```python
from build123d import *

# Parameters (mm, degrees)
F0_R     = 1.294923
F1_DEPTH = 2
F2_W     = 10
F2_H     = 37.403586
F3_DEPTH = 25
F4_W     = 2.4
F4_H     = 37.403586
F5_DEPTH = 20
F6_R     = 1
F7_DEPTH = 25


with BuildPart() as f1:
    # F0 (on Front) → F1 (new body)
    with BuildSketch(Plane.XZ):
        Polygon((23.701793, 0), (0, 23.701793), (-23.701793, 0), (0, -23.701793), align=None)
        with Locations((0, -8)):
            Circle(F0_R, mode=Mode.SUBTRACT)
        with Locations((-8, 0)):
            Circle(F0_R, mode=Mode.SUBTRACT)
        with Locations((8, 0)):
            Circle(F0_R, mode=Mode.SUBTRACT)
        with Locations((0, 8)):
            Circle(F0_R, mode=Mode.SUBTRACT)
    extrude(amount=F1_DEPTH)

    # F2 (on face) → F3 (join)
    with BuildSketch(Plane(origin=(0, 0, 0), x_dir=(-1, 0, 0), z_dir=(0, 1, 0))):
        Rectangle(F2_W, F2_H)
    extrude(amount=F3_DEPTH)

    # F4 (on face) → F5 (cut)
    with BuildSketch(Plane(origin=(0, 25, 0), x_dir=(-1, 0, 0), z_dir=(0, 1, 0))):
        Rectangle(F4_W, F4_H)
    extrude(amount=-F5_DEPTH, mode=Mode.SUBTRACT)

    # F6 (on face) → F7 (cut)
    with BuildSketch(Plane(origin=(-5, 0, 0), x_dir=(0, -1, 0), z_dir=(-1, 0, 0))):
        with Locations((-20, 10)):
            Circle(F6_R)
        with Locations((-10, 10)):
            Circle(F6_R)
        with Locations((-10, 0)):
            Circle(F6_R)
        with Locations((-20, 0)):
            Circle(F6_R)
        with Locations((-20, -10)):
            Circle(F6_R)
        with Locations((-10, -10)):
            Circle(F6_R)
    extrude(amount=-F7_DEPTH, mode=Mode.SUBTRACT)


solid = f1.part
```
The listing builds one solid part. Answer for the finished solid, in the listing's coordinates (mm). A direction names the side the tool comes from. Give positions to 0.01 mm unless a question says otherwise; leave off trailing zeros. Order: outer loops, then holes, each group sorted by start corner. A loop starts at its lowest first (then second) coordinate and runs counter-clockwise, first axis right, second up. Notation, with made-up numbers: M 57,35 L 98,35 A18 ccw 98,42 Z; hole C 15,-19 d9. An arc over 180 degrees is marked long. Put each result on its own line as item: value. Start each with the question number.
Item 1: Which of the six approach directions +Z, -Z, +X, -X, +Y, -Y give full straight-line access (tool end or side, diameter ignored) to faces 4 (the face through (2, 12, -18.702)), 5 (the face through (-0.169, -0.986, 9.284)), 6 (the face through (-3.127, 20.737, -9.324)), 7 (the face through (5, 12, 0)), 8 (the face through (2, 12, 18.702))?
Item 2: The part is cut by section C-C, the plane z = 10. Determine the outline of the cut face in (x, y).
Item 3: For a pull along X with two mould halves and no side action, classify faces 1 (the face through (0, -2, 0)), 2 (the face through (-1.2, 15, 0)), 3 (the face through (-12, -1, -11.7)) as +X half, -X half, draft (parallel to the pull), parting line (faces both ways), or undercut.
Item 4: The part is cut by section A-A, the plane y = 20. State how many separate pieces and enclosed holes the cut face has, and give its area (3 significant figures).
Item 5: The part is cut by section B-B, the plane y = 7. Determine the outline of the cut face in (x, z).
Item 6: The part is cut by section D-D, the plane x = 4. Determine the outline of the cut face in (y, z), and give its area (3 significant figures).
Item 7: Find the intervals of material crossed by line 1 along Z through (x, y) = (3.6, 10); line 2 along X through (y, z) = (14, 0.5); line 3 along Z through (x, y) = (-2, 17.25), in increasing order.
Item 8: Flat-ended cylindrical pins translate along their axes: P1, Ø4, axis at x = -1.5, z = 21, coming from the +Y side; P2, Ø5, axis at x = 1, y = 14, coming from the +Z side; P3, Ø4, axis at y = 17.5, z = -10, coming from the +X side. Find the tip coordinate at first contact, or state that the pin passes through.
Answer key:
1. face 4: -Z, +X, -X, +Y
1. face 5: -Y
1. face 6: +X, -X
1. face 7: +Z, -Z, +X, +Y
1. face 8: +Z, +X, -X, +Y
2. outline: M -13.7,-2 L 13.7,-2 L 13.7,0 L 5,0 L 5,9 L 1.2,9 L 1.2,5 L -1.2,5 L -1.2,9 L -5,9 L -5,0 L -13.7,0 Z; M -5,11 L -1.2,11 L -1.2,19 L -5,19 Z; M -5,21 L -1.2,21 L -1.2,25 L -5,25 Z; M 1.2,11 L 5,11 L 5,19 L 1.2,19 Z; M 1.2,21 L 5,21 L 5,25 L 1.2,25 Z
3. face 1: draft
3. face 2: undercut
3. face 3: -X half
4. separate pieces: 8
4. enclosed holes: 0
4. area: 239 mm²
5. outline: M -5,-18.7 L -1.2,-18.7 L -1.2,18.7 L -5,18.7 Z; M 1.2,-18.7 L 5,-18.7 L 5,18.7 L 1.2,18.7 Z
6. outline: M -2,-19.7 L 0,-19.7 L 0,-18.7 L 25,-18.7 L 25,18.7 L 0,18.7 L 0,19.7 L -2,19.7 Z; hole C 10,-10 d2; hole C 10,0 d2; hole C 10,10 d2; hole C 20,-10 d2; hole C 20,0 d2; hole C 20,10 d2
6. area: 995 mm²
7. line 1: z = -18.7 to -11, -9 to -1, 1 to 9, 11 to 18.7
7. line 2: x = -5 to -1.2, 1.2 to 5
7. line 3: z = -18.7 to 18.7
8. P1: stops at y = 0
8. P2: stops at z = 18.7
8. P3: stops at x = 5
